Part model, mm, in its own coordinate system. Face numbers are marked on the shaded views. A direction names the side the tool comes from. Give positions to 0.01 mm unless a question says otherwise; leave off trailing zeros. Order: outer loops, then holes, each group sorted by start corner. A loop starts at its lowest first (then second) coordinate and runs counter-clockwise, first axis right, second up. Notation, with made-up numbers: M 74,3.25 L 87,3.25 A18 ccw 87,18.25 Z; hole C -27,65.25 d2. An arc over 180 degrees is marked long. Answer as a JSON object with one key per item and string values.
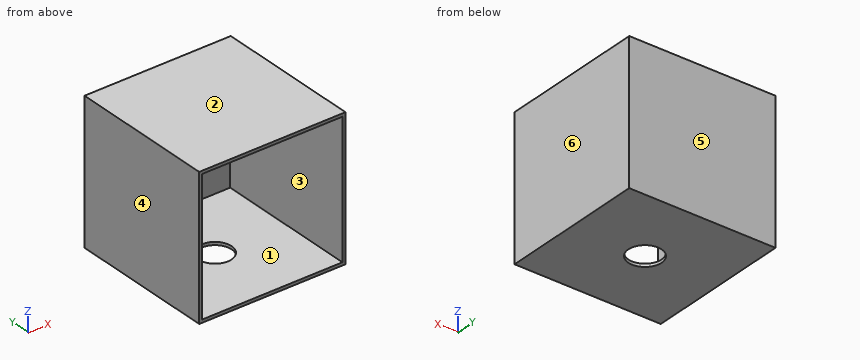
from build123d import *

# Parameters (mm, degrees)
F0_W     = 146
F0_H     = 146
F0_R     = 16.5
F1_DEPTH = 140
F2_T     = -3
F3_DEPTH = 3


with BuildPart() as f1:
    # F0 (on Top) → F1 (new body)
    with BuildSketch(Plane.XY):
        Rectangle(F0_W, F0_H)
        Circle(F0_R, mode=Mode.SUBTRACT)
        Circle(F0_R)
    extrude(amount=F1_DEPTH)

    # F2
    f2_openings = [f1.faces().sort_by_distance(p)[0] for p in [
        (0, -73, 70),
    ]]
    offset(amount=F2_T, openings=f2_openings)

    # F0 (on Top) → F3 (cut)
    with BuildSketch(Plane.XY):
        Circle(F0_R)
    extrude(amount=F3_DEPTH, mode=Mode.SUBTRACT)


solid = f1.part
1. Cut at B-B on y = -22. Give the cut face in (x, z).
Worked answers:
{"outline": "M -73,0 L 73,0 L 73,140 L -73,140 Z; hole M -70,3 L 70,3 L 70,137 L -70,137 Z"}
2. Cut at A-A on x = 0. Give the cut face in (y, z).
Worked answers:
{"outline": "M -73,0 L -16.5,0 L -16.5,3 L -73,3 Z; M -73,137 L 70,137 L 70,3 L 16.5,3 L 16.5,0 L 73,0 L 73,140 L -73,140 Z"}
3. Which spindle directions (+Z, -Z, +X, -X, +Y, -Y) get a long thin tool onto all of the face, cutting with end or side? Do the marked faces 1 and 2. Say none if no direction does.
Worked answers:
{"face 1": "-Y", "face 2": "+Z, +X, -X, +Y, -Y"}
4. Two-plate mould, pull along X, no slides. Class the marked faces 3, 4, 5 and 6: +X half, -X half, draft (parallel to the pull), parting line (faces both ways), or undercut.
Worked answers:
{"face 3": "undercut", "face 4": "-X half", "face 5": "draft", "face 6": "+X half"}
5. Probe line 1 along X through (y, z) = (-4.5, 78); line 2 along Z through (x, y) = (-28, -60); line 3 along Y through (x, z) = (0, 1). List the from-to ranges inside material, lowest first.
Worked answers:
{"line 1": "x = -73 to -70, 70 to 73", "line 2": "z = 0 to 3, 137 to 140", "line 3": "y = -73 to -16.5, 16.5 to 73"}
6. Pin check, flat tips, straight feed: P1, Ø1, axis at x = -20, y = -11.5, coming from the -Z side; P2, Ø5, axis at x = -0.5, z = 47.5, coming from the -Y side. Stop position of each tip, or through.
Worked answers:
{"P1": "stops at z = 0", "P2": "stops at y = 70"}
7. Cut at D-D on y = 0. Give the cut face in (x, z).
Worked answers:
{"outline": "M -73,0 L -16.5,0 L -16.5,3 L -70,3 L -70,137 L 70,137 L 70,3 L 16.5,3 L 16.5,0 L 73,0 L 73,140 L -73,140 Z"}
8. Cut at C-C on z = 54. Give the cut face in (x, y), plus the area to 3 significant figures.
Worked answers:
{"outline": "M -73,-73 L -70,-73 L -70,70 L 70,70 L 70,-73 L 73,-73 L 73,73 L -73,73 Z", "area": "1,300 mm^2"}
